from build123d import *

# Parameters (mm, degrees)
BOSS_EXTRUDE1_DEPTH = 50
FILLET2_R           = 5


with BuildPart() as part:
    # Sketch1 → Boss-Extrude1 (new body)
    with BuildSketch(Plane(origin=(0, 0, 0), x_dir=(1, 0, 0), z_dir=(0, 1, 0))):
        Polygon((0, 0), (72.207221558, 0), (72.207221558, 63.147853309), (54.440853042, 63.147853309), (54.440853042, 16.414579606), (0, 16.414579606), align=None)
    extrude(amount=BOSS_EXTRUDE1_DEPTH)

    # Fillet2
    fillet2_edges = [part.edges().sort_by_distance(p)[0] for p in [
        (0, 25, -16.414579606),
        (54.440853042, 50, -39.781216458),
        (27.220426521, 50, -16.414579606),
        (0, 50, -8.207289803),
        (27.220426521, 0, -16.414579606),
        (54.440853042, 0, -39.781216458),
        (0, 0, -8.207289803),
    ]]
    fillet(fillet2_edges, radius=FILLET2_R)


solid = part.part
Work out the finished part from the listing and answer in its coordinate system (mm). A direction names the side the tool comes from. Round coordinates to 2 decimals unless told otherwise and drop trailing zeros. Order: outer loops, then holes, each group sorted by start corner. A loop starts at its lowest first (then second) coordinate and runs counter-clockwise, first axis right, second up. Notation, with made-up numbers: M 31.5,22 L 39.5,22 A36 ccw 39.5,61 Z; hole C 81,-7.5 d7. An arc over 180 degrees is marked long. One line per item, written item: value.
Q1. A flat-ended cylindrical pin translates along its axis: pin 1 (10 mm diameter, centred on y = 33, z = -28.5, fed in from -X). Find the tip coordinate at first contact, or state that the pin passes through.
Derived:
pin 1: x = 54.44
Q2. Find section D-D on y = 46.5. Write down the section's boundary in (x, z).
Derived:
outline: M 0.23,-11.41 A4.77 ccw 5,-16.18 L 54.67,-16.18 L 54.67,-63.15 L 72.21,-63.15 L 72.21,0 L 0.23,0 Z
Q3. For faces 1 (the face through (30, 25, -16.415)), 2 (the face through (55.87, 1.5, -36.92)), 3 (the face through (31.839, 48.496, -14.989)), determine the directions among +Z, -Z, +X, -X, +Y, -Y from which every point of the face is accessible in a straight line to the end or side of a thin tool.
Derived:
face 1: -Z, -X, +Y, -Y
face 2: -Z, -X, -Y
face 3: -Z, -X, +Y
Q4. Find section A-A on y = 18.5. Write down the section's boundary in (x, z), then the cut area to 3 significant figures.
Derived:
outline: M 0,-11.41 A5 ccw 5,-16.41 L 54.44,-16.41 L 54.44,-63.15 L 72.21,-63.15 L 72.21,0 L 0,0 Z
area: 2,010 mm²
Q5. Find section C-C on z = -26. Write down the section's boundary in (x, y).
Derived:
outline: M 54.44,5 A5 ccw 59.44,0 L 72.21,0 L 72.21,50 L 59.44,50 A5 ccw 54.44,45 Z
Q6. Find section B-B on x = 26.5. Write down the section's boundary in (y, z), then the cut area to 3 significant figures.
Derived:
outline: M 0,-11.41 A5 ccw 5,-16.41 L 45,-16.41 A5 ccw 50,-11.41 L 50,0 L 0,0 Z
area: 810 mm²
Q7. Straight lines are drawn through the part: line 1 (X direction, y = 11, z = -29); line 2 (Z direction, x = 14, y = 28); line 3 (Z direction, x = 3.5, y = 44). For each, find the intervals that lie inside material, in ascending order.
Derived:
line 1: 54.44 to 72.21
line 2: -16.41 to 0
line 3: -16.18 to 0
